Check sheet for the modelled part. Datum: model origin and axes. Units: mm. A direction names the side the tool comes from. Give positions to 0.01 mm unless a question says otherwise; leave off trailing zeros. Order: outer loops, then holes, each group sorted by start corner. A loop starts at its lowest first (then second) coordinate and runs counter-clockwise, first axis right, second up. Notation, with made-up numbers: (-4.75, -10) -> (26.25, -10) arc R21 ccw to (26.25, 3) -> close; hole circle Ø6 at (6, 77). An arc over 180 degrees is marked (long way). Write each question's results on one line, items separated by ' | '.
Autodesk Inventor part; units mm, degrees
ref_plane "Work Plane1" through (0, 0, -15) normal (0, 0, 1) x (1, 0, 0)
ref_plane "YZ Plane" through (0, 0, 0) normal (1, 0, 0) x (0, 1, 0)
ref_plane "XZ Plane" through (0, 0, 0) normal (0, 1, 0) x (-1, 0, 0)
sketch "Sketch1" plane through (0, 0, 0) normal (0, 0, 1) x (1, 0, 0)
  line L0 (0, 0) -> (25, 0)
  line L1 (25, 0) -> (25, 40)
  line L2 (25, 40) -> (0, 40)
  line L3 (0, 40) -> (0, 0)
  dimension "d1" = 25
  dimension "d2" = 40
  dimension "d3" = 25
extrude "Extrusion1" add sketch "Sketch1" against normal blind 30
sketch "Sketch2" plane through (25, 0, 0) normal (1, 0, 0) x (0, 0, -1)
  line L0 (0, 0) -> (30, 0)
  circle A0 centre (15, 6.56) radius 2.46
extrude "Extrusion2" cut sketch "Sketch2" against normal blind 30
sketch "Sketch3" plane through (0, 0, 0) normal (-1, 0, 0) x (0, 0, 1)
  line L0 (0, 0) -> (-30, 0)
  line L1 (-25.05, 0) -> (-4.95, 0)
  line L2 (-4.95, 0) -> (-4.95, 33.12)
  line L3 (-4.95, 33.12) -> (-25.05, 33.12)
  line L4 (-25.05, 33.12) -> (-25.05, 0)
  dimension "d11" = 20.1
extrude "Extrusion3" cut sketch "Sketch3" against normal blind 20
sketch "Sketch4" plane through (0, 0, 0) normal (0, -1, 0) x (1, 0, 0)
  line L0 (20, -4.95) -> (20, -25.05)
  line L1 (20, -15) -> (25, -15)
  line L2 (25, 0) -> (25, -30)
  line L3 (20, -8.025) -> (25, -8.025)
  line L4 (25, -8.025) -> (25, -21.975)
  line L5 (25, -21.975) -> (20, -21.975)
  line L6 (20, -21.975) -> (20, -8.025)
  line L7 (20, -8.025) -> (25, -21.975) construction
  line L8 (25, -8.025) -> (20, -21.975) construction
  line L9 (25, -12.54) -> (25, -17.46)
  point P0 (0, 0)
  point P1 (22.5, -15)
  dimension "d14" = 13.95
extrude "Extrusion4" add sketch "Sketch4" along normal blind 15
sketch "Sketch5" plane through (20, 0, 0) normal (-1, 0, 0) x (0, 0, 1)
  circle A0 centre (-15, 6.56) radius 2.46
  circle A1 centre (-15, 6.56) radius 4.7025
  circle A2 centre (-15, 6.56) radius 2.46
  circle A3 centre (-15, 6.56) radius 2.46
  point P0 (0, 0)
  dimension "d17" = 9.405
extrude "Extrusion5" cut sketch "Sketch5" against normal blind 2.1
sketch "Sketch6" plane through (25, 0, 0) normal (1, 0, 0) x (0, 0, -1)
  circle A0 centre (15, 6.56) radius 4.7025
  line L0 (15, 6.56) -> (15, 23.56)
  circle A1 centre (15, 23.56) radius 2.46
  point P0 (0, 0)
  dimension "d20" = 17
  dimension "d21" = 4.92
extrude "Extrusion6" cut sketch "Sketch6" against normal blind 10 contours A1
sketch "Sketch7" plane through (20, 0, 0) normal (-1, 0, 0) x (0, 0, 1)
  circle A0 centre (-15, 23.56) radius 2.46
  circle A1 centre (-15, 23.56) radius 4.7025
  point P0 (0, 0)
  dimension "d24" = 9.405
extrude "Extrusion7" cut sketch "Sketch7" against normal blind 2.1
sketch "Sketch9" plane through (25, 0, 0) normal (1, 0, 0) x (0, 0, -1)
  circle A0 centre (15, 6.56) radius 2.46
  circle A1 centre (15, 6.56) radius 2.46
  circle A2 centre (15, 23.56) radius 2.46
  circle A3 centre (15, 23.56) radius 2.46
  line L0 (30, 40) -> (30, 0)
  line L1 (30, 0) -> (30, 40)
  line L2 (30, 40) -> (0, 40)
  line L3 (0, 40) -> (0, 0)
  line L4 (0, 0) -> (8.025, 0)
  line L5 (21.975, 0) -> (21.975, -15)
  line L6 (21.975, -15) -> (8.025, -15)
  line L7 (8.025, -15) -> (8.025, 0)
  line L8 (0, 0) -> (8.025, 0)
  line L9 (21.975, 0) -> (30, 0)
extrude "Extrusion8" add sketch "Sketch9" along normal blind 5
sketch "Sketch10" plane through (0, 40, 0) normal (0, 1, 0) x (1, 0, 0)
  line L0 (0, 30) -> (30, 30)
  line L1 (30, 0) -> (0, 0)
  line L2 (0, 30) -> (30, 30)
  line L3 (30, 30) -> (30, 0)
  line L4 (30, 0) -> (0, 0)
  line L5 (0, 0) -> (0, 30)
extrude "Extrusion9" add sketch "Sketch10" along normal blind 30
sketch "Sketch12" plane through (30, 0, 0) normal (1, 0, 0) x (0, 0, -1)
  circle A0 centre (15, 6.56) radius 2.46
  line L0 (15, 6.56) -> (15, 15.06)
  circle A1 centre (15, 15.06) radius 2.525
  point P0 (0, 0)
  dimension "d31" = 8.5
  dimension "d33" = 5.05
extrude "Extrusion10" cut sketch "Sketch12" against normal blind 30 contours A1
sketch "Sketch14" plane through (0, 0, 0) normal (0, 0, 1) x (1, 0, 0)
  line L0 (30, 70) -> (0, 70)
  line L1 (0, 70) -> (0, 85)
  line L2 (-15, 100) -> (-23, 100)
  line L3 (30, 0) -> (30, 70)
  line L4 (30, 109) -> (30, 70)
  arc A0 (0, 85) -> (-15, 100) centre (-15, 85) ccw
  line L5 (30, 105) -> (30, 100)
  line L6 (-23, 124) -> (15, 124)
  line L7 (-19, 122) -> (-23, 124)
  line L8 (-19, 122) -> (-15, 112)
  line L9 (-19, 102) -> (-23, 100)
  line L10 (-19, 102) -> (-15, 112)
  line L11 (30, 109) -> (15, 124)
  point P0 (0, 0)
  point P1 (0, 100)
  dimension "d47" = 30
  dimension "d54" = 15
extrude "Extrusion12" add sketch "Sketch14" against normal blind 30
sketch "Sketch15" plane through (0, 0, -25.05) normal (-1, 0, 0) x (0, 0, 1)
  line L0 (0, 33.12) -> (20.1, 33.12)
  line L1 (20.1, 33.12) -> (20.1, 0)
  line L2 (0, 33.12) -> (20.1, 33.12)
  line L3 (20.1, 33.12) -> (20.1, 31.1)
  line L4 (20.1, 31.1) -> (0, 31.1)
  line L5 (0, 31.1) -> (0, 33.12)
  point P0 (25.05, 0)
  dimension "d57" = 2.02
extrude "Extrusion13" add sketch "Sketch15" against normal blind 20
sketch "Sketch19" plane through (0, 0, 0) normal (0, 0, 1) x (1, 0, 0)
  arc A0 (0, 85) -> (-15, 100) centre (-15, 85) ccw
  arc A1 (0, 85) -> (-15, 100) centre (-15, 85) ccw
  line L0 (-15, 100) -> (-23, 100)
  line L1 (-15, 100) -> (-23, 100)
  line L2 (-23, 100) -> (-19, 102)
  line L3 (-23, 100) -> (-19, 102)
  line L4 (-19, 102) -> (-15, 112)
  line L5 (-19, 102) -> (-15, 112)
  line L6 (-15, 112) -> (-19, 122)
  line L7 (-15, 112) -> (-19, 122)
  line L8 (-19, 122) -> (-23, 124)
  line L9 (-19, 122) -> (-23, 124)
  line L10 (-23, 124) -> (15, 124)
  line L11 (-23, 124) -> (15, 124)
  line L12 (15, 124) -> (30, 109)
  line L13 (15, 124) -> (30, 109)
  line L14 (30, 109) -> (30, 85)
  line L15 (30, 0) -> (30, 109)
  line L16 (0, 85) -> (30, 85)
  point P0 (0, 0)
extrude "Extrusion14" add sketch "Sketch19" along normal blind 45
ref_plane "Work Plane1" through (0, 0, -15) normal (0, 0, 1) x (1, 0, 0)
mirror "Mirror1" about plane through (0, 0, -15) normal (0, 0, 1) of "Extrusion14"
properties part number "20mm_x_120mm"
1. Gauge pin test, flat ends, axial feed: pin 1 Ø4 at (y, z) = (15.06, -15) entering from -X; pin 2 Ø10 at (x, y) = (12, 20) entering from +Z; pin 3 Ø24 at (x, z) = (11, -50.5) entering from -Y; pin 4 Ø5 at (x, y) = (27, -7) entering from -Z (3 decimals). Record the tip position at first contact, or that the pin passes through.
Verdict:
pin 1: passes through | pin 2: stops at z = 0 | pin 3: stops at y = 85 | pin 4: stops at z = -21.975
2. Section check A-A on z = -15. Give the number of separate pieces and of enclosed holes in the cut face, then the cut area to 3 significant figures.
Verdict:
separate pieces: 4 | enclosed holes: 0 | area: 3,440 mm^2
3. Section check B-B on y = 15.06. Record the cut outline in (x, z) (3 decimals), then the cut area to 4 significant figures.
Verdict:
outline: (0, -30) -> (30, -30) -> (30, -17.525) -> (20, -17.525) -> (20, -25.05) -> (0, -25.05) -> close; (0, -4.95) -> (20, -4.95) -> (20, -12.475) -> (30, -12.475) -> (30, 0) -> (0, 0) -> close | area: 447.5 mm^2
4. Access from +Z, -Z, +X, -X, +Y, -Y to the whole of each face (thin tool, end or side, straight path). Record for faces 1 (the flat face through (-19, 100, -14)), 2 (the flat face through (15, 0, -3)), 3 (the flat face through (-17, 107, -14)), 4 (the flat face through (15, 43, -30)).
Verdict:
face 1: +Z, -Z, -X, -Y | face 2: +Z, +X, -X, -Y | face 3: +Z, -Z, -X | face 4: -Z, +X, -X, -Y
5. Section check D-D on x = 11.5. Record the cut outline in (y, z).
Verdict:
outline: (0, -30) -> (85, -30) -> (85, -75) -> (124, -75) -> (124, 45) -> (85, 45) -> (85, 0) -> (0, 0) -> (0, -4.95) -> (31.1, -4.95) -> (31.1, -25.05) -> (0, -25.05) -> close
6. Section check C-C on z = -62. Record the cut outline in (x, y), then the cut area to 3 significant figures.
Verdict:
outline: (-23, 100) -> (-15, 100) arc R15 cw to (0, 85) -> (30, 85) -> (30, 109) -> (15, 124) -> (-23, 124) -> (-19, 122) -> (-15, 112) -> (-19, 102) -> close | area: 1,530 mm^2
7. Material ranges on probe 1 along Z at (x, y) = (1, 10); probe 2 along Y at (x, z) = (27, -15) (3 decimals); probe 3 along Z at (x, y) = (26.5, 23.56), recorded low to high. Write a range as from..to.
Verdict:
probe 1: z = -30..-25.05, -4.95..0 | probe 2: y = -15..4.1, 9.02..12.535, 17.585..21.1, 26.02..112 | probe 3: z = -30..-17.46, -12.54..0
8. Mould release check, pull along Y, two halves, no side actions. Record for faces 5 (the cylindrical face through (25.07, 15.171, -12.477)), 6 (the flat face through (22.1, 21.5, -13)), 7 (the cylindrical face through (-4.28, 95.49, -14.16)), 8 (the flat face through (30, 60, -14)): +Y half, -Y half, draft (parallel to the pull), parting line (faces both ways), or undercut.
Verdict:
face 5: undercut | face 6: undercut | face 7: -Y half | face 8: draft
